Input: part model. Units: mm. Frame: model coordinates. A direction names the side the tool comes from. Give positions to 0.01 mm unless a question says otherwise; leave off trailing zeros. Write each loop counter-clockwise with the first axis right and the second up, starting at its lowest first coordinate (ties: lowest second). Pieces come first, ordered by that corner, then holes. Notation, with made-up numbers: (4, -20) -> (11, -20) arc R26 ccw to (11, 11) -> close; hole circle Ø11 at (12, 72). An arc over 180 degrees is marked (long way). Answer as a JSON object with one key per item and string values. Group by question number.
from build123d import *

# Parameters (mm, degrees)
SKETCH1_W               = 20
SKETCH1_H               = 28
BOSS_EXTRUDE1_DEPTH     = 28
SKETCH2_W               = 24
SKETCH2_H               = 20
CUT_EXTRUDE1_DEPTH      = 6
CUT_EXTRUDE1_DEPTH_BACK = 6
CUT_EXTRUDE2_DEPTH      = 20
FILLET1_R               = 2
SKETCH4_R               = 1.9
CUT_EXTRUDE3_DEPTH      = 10
SKETCH5_R               = 1.9
CUT_EXTRUDE4_DEPTH      = 5
FILLET2_R               = 2
FILLET3_R               = 3


with BuildPart() as part:
    # Sketch1 → Boss-Extrude1 (new body)
    with BuildSketch(Plane.XY):
        Rectangle(SKETCH1_W, SKETCH1_H)
    extrude(amount=BOSS_EXTRUDE1_DEPTH)

    # Sketch2 → Cut-Extrude1 (cut, two sides)
    with BuildSketch(Plane.ZY) as cut_extrude1_sk:
        with Locations((16, -4)):
            Rectangle(SKETCH2_W, SKETCH2_H)
    extrude(amount=CUT_EXTRUDE1_DEPTH, mode=Mode.SUBTRACT)
    extrude(cut_extrude1_sk.sketch, amount=-CUT_EXTRUDE1_DEPTH_BACK, mode=Mode.SUBTRACT)

    # Sketch3 → Cut-Extrude2 (cut)
    with BuildSketch(Plane.ZY.offset(10)):
        Polygon((28, 14), (4, -14), (28, -14), align=None)
    extrude(amount=-CUT_EXTRUDE2_DEPTH, mode=Mode.SUBTRACT)

    # Fillet1
    fillet1_edges = [part.edges().sort_by_distance(p)[0] for p in [
        (0, 14, 28),
    ]]
    fillet(fillet1_edges, radius=FILLET1_R)

    # Sketch4 → Cut-Extrude3 (cut)
    with BuildSketch(Plane(origin=(0, 14, 0), x_dir=(1, 0, 0), z_dir=(0, 1, 0))):
        with Locations((0, -11)):
            Circle(SKETCH4_R)
        with Locations((0, -18)):
            Circle(SKETCH4_R)
    extrude(amount=-CUT_EXTRUDE3_DEPTH, mode=Mode.SUBTRACT)

    # Sketch5 → Cut-Extrude4 (cut, through all)
    with BuildSketch(Plane.XY.offset(4)):
        with Locations((0, -2)):
            Circle(SKETCH5_R)
        with Locations((0, -10)):
            Circle(SKETCH5_R)
    extrude(amount=-CUT_EXTRUDE4_DEPTH, mode=Mode.SUBTRACT)

    # Fillet2
    fillet2_edges = [part.edges().sort_by_distance(p)[0] for p in [
        (0, -14, 0),
    ]]
    fillet(fillet2_edges, radius=FILLET2_R)

    # Fillet3
    fillet3_edges = [part.edges().sort_by_distance(p)[0] for p in [
        (0, 14, 0),
    ]]
    fillet(fillet3_edges, radius=FILLET3_R)


solid = part.part
1. Section C-C (x = -2.25). Return the cut outline in (y, z).
2. Reachability of faces 5 (the face through (0.14, 13.1, 0.86)), 6 (the face through (-1.4, 6, 12.5)) from +Z, -Z, +X, -X, +Y, -Y: full face, straight path, thin tool, end or side. Return the list, or none.
3. Section D-D (x = 1.25). Return the cut outline in (y, z), plus the area to 3 significant figures.
4. Section A-A (z = 18). Return the cut outline in (x, y), plus the area to 3 significant figures.
5. Line query: line 1 (X direction, y = 11.5, z = 11); line 2 (Z direction, x = 0, y = 11.25); line 3 (X direction, y = -5, z = 10). Output: solid intervals per line, ascending.
6. Section B-B (y = -9.25). Return the cut outline in (x, z).
7. Mould query, pull axis X, two halves, no side actions, for faces 1 (the face through (-0.1, 14, 13.2)), 2 (the face through (6, -2, 11)), 3 (the face through (-0.247, 10.056, 16.116)), 4 (the face through (-10, 3, 10)). Classes: pulls with the +X half, pulls with the -X half, needs draft (parallel to the pull), parting line crosses it, or undercut.
8. Contact query for flat-ended pins moving along their axis: pin 1 Ø3.5 at (x, z) = (0, 18) entering from -Y; pin 2 Ø8 at (x, y) = (5, -5) entering from +Z; pin 3 Ø4.5 at (x, y) = (0, -2) entering from +Z; pin 4 Ø8 at (x, y) = (-6, -3.5) entering from +Z. Output: stop coordinate, or through.
Working result:
{
 "1": {"outline": "(-14, 2) arc R2 ccw to (-12, 0) -> (11, 0) arc R3 ccw to (14, 3) -> (14, 23.65) arc R2 ccw to (10.7, 25.17) -> (6, 21.14) -> (6, 4) -> (-14, 4) -> close"},
 "2": {"face 5": "-Z, +X, -X, +Y", "face 6": "+Z, -Y"},
 "3": {"outline": "(-14, 2) arc R2 ccw to (-12, 0) -> (-11.43, 0) -> (-11.43, 4) -> (-14, 4) -> close; (-8.57, 0) -> (-3.43, 0) -> (-3.43, 4) -> (-8.57, 4) -> close; (-0.57, 0) -> (11, 0) arc R3 ccw to (14, 3) -> (14, 9.57) -> (6, 9.57) -> (6, 4) -> (-0.57, 4) -> close; (6, 12.43) -> (14, 12.43) -> (14, 16.57) -> (6, 16.57) -> close; (6, 19.43) -> (14, 19.43) -> (14, 23.65) arc R2 ccw to (10.7, 25.17) -> (6, 21.14) -> close", "area": "201 mm^2"},
 "4": {"outline": "(-10, 2.33) -> (-6, 2.33) -> (-6, 6) -> (-1.9, 6) -> (-1.9, 14) -> (-10, 14) -> close; (1.9, 6) -> (6, 6) -> (6, 2.33) -> (10, 2.33) -> (10, 14) -> (1.9, 14) -> close", "area": "159 mm^2"},
 "5": {"line 1": "x = -10 to -1.9, 1.9 to 10", "line 2": "z = 0.01 to 9.1, 12.9 to 16.1, 19.9 to 25.51", "line 3": "x = -10 to -6, 6 to 10"},
 "6": {"outline": "(-10, 0) -> (-1.75, 0) -> (-1.75, 4) -> (-6, 4) -> (-6, 8.07) -> (-10, 8.07) -> close; (1.75, 0) -> (10, 0) -> (10, 8.07) -> (6, 8.07) -> (6, 4) -> (1.75, 4) -> close"},
 "7": {"face 1": "needs draft", "face 2": "undercut", "face 3": "undercut", "face 4": "pulls with the -X half"},
 "8": {"pin 1": "passes through", "pin 2": "stops at z = 15.03", "pin 3": "stops at z = 4", "pin 4": "stops at z = 16.43"}
}
